Geometry: final body of the model. Coordinates: model frame, mm. A direction names the side the tool comes from. Round coordinates to 2 decimals unless told otherwise and drop trailing zeros. Loops run counter-clockwise (first coordinate to the right, second up) from the corner with the lowest first, then second, coordinate; pieces in that order, holes last. Notation, with made-up numbers: M 2,-8.75 L 9,-8.75 A27 cw 9,27.25 Z; hole C 14,41.25 d2. An arc over 180 degrees is marked long. Return JSON: item names as keys, results as strings.
from build123d import *

# Parameters (mm, degrees)
SKETCH1_W            = 12.7
SKETCH1_H            = 12.7
BOSS_EXTRUDE1_DEPTH  = 44.45
SKETCH2_R            = 6.35
BOSS_EXTRUDE2_DEPTH  = 19.05
SKETCH3_W            = 25.4
SKETCH3_H            = 12.7
BOSS_EXTRUDE3_DEPTH  = 28.652
BOSS_EXTRUDE4_START  = 19.05
SKETCH4_W            = 19.05
SKETCH4_H            = 12.7
BOSS_EXTRUDE4_DEPTH  = 9.602
CUT_EXTRUDE1_START   = -41.352
CUT_EXTRUDE1_DEPTH   = 41.352
BOSS_EXTRUDE5_START  = -31.75
SKETCH2_2_R          = 6.35
BOSS_EXTRUDE5_DEPTH  = 19.05
CUT_EXTRUDE2_START   = -4
SKETCH6_R            = 1.395358984
CUT_EXTRUDE2_DEPTH   = 4
CUT_EXTRUDE4_START   = -6.35
SKETCH6_2_R          = 1.395358984
CUT_EXTRUDE4_DEPTH   = 6.35
SKETCH8_W            = 41.352
SKETCH8_H            = 25.4
BOSS_EXTRUDE6_DEPTH  = 19.05
BOSS_EXTRUDE7_START  = -12.7
SKETCH8_2_W          = 41.352
SKETCH8_2_H          = 25.4
BOSS_EXTRUDE7_DEPTH  = 10.668
SKETCH9_W            = 20.066
SKETCH9_H            = 39.878
CUT_EXTRUDE5_DEPTH   = 30.48
SKETCH11_W           = 16.764
SKETCH11_H           = 2.667
SKETCH11_W_2         = 10.872
SKETCH11_H_2         = 3.65
SKETCH11_W_3         = 1.618
BOSS_EXTRUDE8_DEPTH  = 8.622
BOSS_EXTRUDE9_START  = 8.622
SKETCH11_3_W         = 16.764
SKETCH11_3_H         = 2.667
SKETCH11_3_W_2       = 10.872
SKETCH11_3_H_2       = 3.65
SKETCH11_3_W_3       = 1.618
BOSS_EXTRUDE9_DEPTH  = 8.89
BOSS_EXTRUDE10_START = 17.512
BOSS_EXTRUDE10_DEPTH = 6.35
SKETCH12_W           = 15.5
SKETCH12_H           = 7.5
CUT_EXTRUDE7_DEPTH   = 83.562249267
CUT_EXTRUDE8_START   = -1.905
CUT_EXTRUDE8_DEPTH   = 81.657249267


# Read off the part's stored shape, not the designer's step: Cut-Extrude1
with BuildPart() as part:
    # Sketch1 → Boss-Extrude1 (new body)
    with BuildSketch(Plane.XY):
        Rectangle(SKETCH1_W, SKETCH1_H)
    extrude(amount=BOSS_EXTRUDE1_DEPTH)

    # Sketch2 → Boss-Extrude2 (add)
    with BuildSketch(Plane(origin=(6.35, 0, 0), x_dir=(0, 0, -1), z_dir=(1, 0, 0))):
        with Locations(Location((-38.1, 0, 0), (0, 0, 180))):
            Circle(SKETCH2_R)
    extrude(amount=BOSS_EXTRUDE2_DEPTH)

    # Sketch3 → Boss-Extrude3 (add)
    with BuildSketch(Plane.ZY.offset(6.35)):
        with Locations((12.7, 0)):
            Rectangle(SKETCH3_W, SKETCH3_H)
    extrude(amount=BOSS_EXTRUDE3_DEPTH)

    # Sketch4 → Boss-Extrude4 (add)
    with BuildSketch(Plane.ZY.offset(6.35).offset(BOSS_EXTRUDE4_START)):
        with Locations((34.925, 0)):
            Rectangle(SKETCH4_W, SKETCH4_H)
    extrude(amount=BOSS_EXTRUDE4_DEPTH)

    # Cut-Extrude1 outline → Cut-Extrude1 (cut)
    with BuildSketch(Plane(origin=(6.35, 0, 0), x_dir=(0, 0, -1), z_dir=(1, 0, 0)).offset(CUT_EXTRUDE1_START)):
        with BuildLine():
            ThreePointArc((-44.45, 0), (-42.590128061, 4.490128061), (-38.1, 6.35))
            Line((-38.1, 6.35), (-44.45, 6.35))
            Line((-44.45, 6.35), (-44.45, 0))
        make_face()
        with BuildLine():
            Line((-44.45, -6.35), (-38.1, -6.35))
            ThreePointArc((-38.1, -6.35), (-42.590128061, -4.490128061), (-44.45, 0))
            Line((-44.45, 0), (-44.45, -6.35))
        make_face()
    extrude(amount=CUT_EXTRUDE1_DEPTH, mode=Mode.SUBTRACT)

    # Sketch2<2> → Boss-Extrude5 (add)
    with BuildSketch(Plane(origin=(6.35, 0, 0), x_dir=(0, 0, -1), z_dir=(1, 0, 0)).offset(BOSS_EXTRUDE5_START)):
        with Locations(Location((-38.1, 0, 0), (0, 0, 90))):
            Circle(SKETCH2_2_R)
    extrude(amount=BOSS_EXTRUDE5_DEPTH)

    # Sketch6 → Cut-Extrude2 (cut)
    with BuildSketch(Plane.ZY.offset(35.002).offset(CUT_EXTRUDE2_START)):
        with BuildLine():
            Line((27.722, -3.706), (13.572, -3.706))
            ThreePointArc((13.572, -3.706), (9.772, 0.094), (13.572, 3.894))
            Line((13.572, 3.894), (27.722, 3.894))
            ThreePointArc((27.722, 3.894), (30.88427766, 4.407167019), (33.722, 5.894))
            ThreePointArc((33.722, 5.894), (45.322, 0.094), (33.722, -5.706))
            ThreePointArc((33.722, -5.706), (30.88427766, -4.219167019), (27.722, -3.706))
        make_face()
        with Locations(Location((17.572, 0.094, 0), (0, 0, 270))):
            Circle(SKETCH6_R, mode=Mode.SUBTRACT)
        with Locations(Location((13.572, 0.094, 0), (0, 0, 270))):
            Circle(SKETCH6_R, mode=Mode.SUBTRACT)
    extrude(amount=CUT_EXTRUDE2_DEPTH, mode=Mode.SUBTRACT)

    # Sketch6<2> → Cut-Extrude4 (cut)
    with BuildSketch(Plane.ZY.offset(35.002).offset(CUT_EXTRUDE4_START)):
        with Locations(Location((13.572, 0.094, 0), (0, 0, 270))):
            Circle(SKETCH6_2_R)
        with Locations(Location((17.572, 0.094, 0), (0, 0, 270))):
            Circle(SKETCH6_2_R)
    extrude(amount=CUT_EXTRUDE4_DEPTH, mode=Mode.SUBTRACT)

    # Sketch8 → Boss-Extrude6 (add)
    with BuildSketch(Plane.XZ.offset(6.35)):
        with Locations((-14.326, 12.7)):
            Rectangle(SKETCH8_W, SKETCH8_H)
    extrude(amount=BOSS_EXTRUDE6_DEPTH)

    # Sketch8<2> → Boss-Extrude7 (add)
    with BuildSketch(Plane.XZ.offset(6.35).offset(BOSS_EXTRUDE7_START)):
        with Locations((-14.326, 12.7)):
            Rectangle(SKETCH8_2_W, SKETCH8_2_H)
    extrude(amount=-BOSS_EXTRUDE7_DEPTH)

    # Sketch9 → Cut-Extrude5 (cut)
    with BuildSketch(Plane(origin=(6.35, 0, 0), x_dir=(0, 0, -1), z_dir=(1, 0, 0))):
        with Locations((-12.7, -2.921)):
            Rectangle(SKETCH9_W, SKETCH9_H)
    extrude(amount=-CUT_EXTRUDE5_DEPTH, mode=Mode.SUBTRACT)

    # Sketch11 → Boss-Extrude8 (add)
    with BuildSketch(Plane(origin=(0, 17.018, 0), x_dir=(1, 0, 0), z_dir=(0, 1, 0))):
        with Locations((-14.13, -24.0665)):
            Rectangle(SKETCH11_W, SKETCH11_H)
        Polygon((-22.512, -25.4), (-22.512, -22.733), (-24.13, -22.733), (-35.002, -22.733), (-35.002, -25.4), align=None)
        with Locations((-29.566, -20.908)):
            Rectangle(SKETCH11_W_2, SKETCH11_H_2)
        with Locations((-23.321, -20.908)):
            Rectangle(SKETCH11_W_3, SKETCH11_H_2)
    extrude(amount=BOSS_EXTRUDE8_DEPTH)

    # Sketch11<3> → Boss-Extrude9 (add)
    with BuildSketch(Plane(origin=(0, 17.018, 0), x_dir=(1, 0, 0), z_dir=(0, 1, 0)).offset(BOSS_EXTRUDE9_START)):
        with Locations((-14.13, -24.0665)):
            Rectangle(SKETCH11_3_W, SKETCH11_3_H)
        with Locations((-29.566, -20.908)):
            Rectangle(SKETCH11_3_W_2, SKETCH11_3_H_2)
        Polygon((-22.512, -25.4), (-22.512, -22.733), (-24.13, -22.733), (-35.002, -22.733), (-35.002, -25.4), align=None)
        with Locations((-23.321, -20.908)):
            Rectangle(SKETCH11_3_W_3, SKETCH11_3_H_2)
    extrude(amount=BOSS_EXTRUDE9_DEPTH)

    # Sketch11<4> → Boss-Extrude10 (add)
    with BuildSketch(Plane(origin=(0, 17.018, 0), x_dir=(1, 0, 0), z_dir=(0, 1, 0)).offset(BOSS_EXTRUDE10_START)):
        with BuildLine():
            Line((-5.748, -22.733), (-5.748, -12.733))
            ThreePointArc((-5.748, -12.733), (-6.313107632, -9.707422748), (-7.932232333, -7.089809417))
            ThreePointArc((-7.932232333, -7.089809417), (-9.3675, -7.022587953), (-9.434721465, -8.457855619))
            ThreePointArc((-9.434721465, -8.457855619), (-14.13, -19.083), (-18.825278535, -8.457855619))
            ThreePointArc((-18.825278535, -8.457855619), (-18.8925, -7.022587953), (-20.327767667, -7.089809417))
            ThreePointArc((-20.327767667, -7.089809417), (-21.946892368, -9.707422748), (-22.512, -12.733))
            Line((-22.512, -12.733), (-22.512, -19.083))
            Line((-22.512, -19.083), (-22.512, -22.733))
            Line((-22.512, -22.733), (-5.748, -22.733))
        make_face()
    extrude(amount=-BOSS_EXTRUDE10_DEPTH)

    # Sketch12 → Cut-Extrude7 (cut, through all)
    with BuildSketch(Plane.ZY.offset(35.002)):
        with Locations((12.733, -17.61)):
            Rectangle(SKETCH12_W, SKETCH12_H)
    extrude(amount=-CUT_EXTRUDE7_DEPTH, mode=Mode.SUBTRACT)

    # Sketch12<3> → Cut-Extrude8 (cut, through all)
    with BuildSketch(Plane.ZY.offset(35.002).offset(CUT_EXTRUDE8_START)):
        Polygon((13.737, 8.094), (22.387, 8.094), (22.387, 4.386), (3.079, 4.386), (3.079, 8.094), (11.729, 8.094), (11.729, 10.094), (13.737, 10.094), align=None)
    extrude(amount=-CUT_EXTRUDE8_DEPTH, mode=Mode.SUBTRACT)


solid = part.part
Q1. Pull-direction query (Z, two-part tool) for faces 1 (the cylindrical face through (-29.81, 0.4, 16.21)), 2 (the flat face through (-29, 26, 19.083)), 3 (the flat face through (-30, -6.35, 32)); classes: pulls with the +Z half, pulls with the -Z half, needs draft (parallel to the pull), parting line crosses it, or undercut.
Determined:
{"face 1": "undercut", "face 2": "pulls with the -Z half", "face 3": "needs draft"}
Q2. Reachability of faces 4 (the cylindrical face through (-29.81, 0.4, 12.21)), 5 (the flat face through (-22.512, 31, 16)), 6 (the flat face through (-29, 9, 13.737)) from +Z, -Z, +X, -X, +Y, -Y: full face, straight path, thin tool, end or side. Return the list, or none.
Determined:
{"face 4": "-X", "face 5": "-Z, -X, +Y", "face 6": "+X"}
Q3. Section query A-A (x = -14.13). Output: boundary loops of the cut face in (y, z), plus the area to 3 significant figures.
Determined:
{"outline": "M -25.4,0 L 17.02,0 L 17.02,2.67 L -22.86,2.67 L -22.86,22.73 L 28.18,22.73 L 28.18,19.08 L 34.53,19.08 L 34.53,25.4 L -25.4,25.4 Z; C 0,38.1 d12.7", "area": "474 mm^2"}
Q4. Pin query (flat end, axial travel): pin 1 (1 mm diameter, centred on x = -28, y = 9, fed in from +Z); pin 2 (6.5 mm diameter, centred on y = 6, z = 12, fed in from +X); pin 3 (12 mm diameter, centred on y = 18, z = 34.5, fed in from +X); pin 4 (5 mm diameter, centred on y = 16, z = 23.5, fed in from +X). Return the tip coordinate at first contact, or that it passes through.
Determined:
{"pin 1": "stops at z = 25.4", "pin 2": "stops at x = -24.13", "pin 3": "passes through", "pin 4": "stops at x = 6.35"}
Q5. Section query B-B (y = -17). Output: boundary loops of the cut face in (x, z), plus the area to 3 significant figures.
Determined:
{"outline": "M -35,0 L 6.35,0 L 6.35,2.67 L -24.13,2.67 L -24.13,4.98 L -35,4.98 Z; M -35,20.48 L -24.13,20.48 L -24.13,22.73 L 6.35,22.73 L 6.35,25.4 L -35,25.4 Z", "area": "270 mm^2"}
Q6. Material intervals for L1, parallel to X at y = -4, z = 30; L2, parallel to Y at x = -12.5, z = 22; L3, parallel to Z at x = -15.5, y = -13, sorted ascending.
Determined:
{"L1": "x = -35 to -25.4, -6.35 to 6.35", "L2": "y = -25.4 to -22.86, 28.18 to 34.53", "L3": "z = 0 to 2.67, 22.73 to 25.4"}
Q7. Section query C-C (y = -9). Output: boundary loops of the cut face in (x, z), plus the area to 3 significant figures.
Determined:
{"outline": "M -35,0 L 6.35,0 L 6.35,2.67 L -24.13,2.67 L -24.13,22.73 L 6.35,22.73 L 6.35,25.4 L -35,25.4 Z", "area": "439 mm^2"}
Q8. Section query D-D (z = 28.5). Output: boundary loops of the cut face in (x, y), plus the area to 3 significant figures.
Determined:
{"outline": "M -35,-6.35 L -25.4,-6.35 L -25.4,6.35 L -35,6.35 L -35,3.92 L -31,3.92 L -31,-3.74 L -35,-3.74 Z; M -6.35,-6.35 L 6.35,-6.35 L 6.35,6.35 L -6.35,6.35 Z", "area": "253 mm^2"}
